```python
from build123d import *

# Parameters (mm, degrees)
SKETCH2_R          = 70
CUT_EXTRUDE1_DEPTH = 10
SKETCH3_R          = 20
CUT_EXTRUDE2_DEPTH = 121
SKETCH4_W          = 19.454924149
SKETCH4_H          = 15
CUT_EXTRUDE3_DEPTH = 121


with BuildPart() as part:
    # Sketch1 → Revolve1 (revolve)
    with BuildSketch(Plane.XY):
        Polygon((0, 65), (160, 65), (160, 40), (110, 40), (110, -40), (160, -40), (160, -65), (0, -65), align=None)
    revolve(axis=Axis((0, 93.810810811, 0), (0, -1, 0)))

    # Sketch2 → Cut-Extrude1 (cut)
    with BuildSketch(Plane(origin=(0, 65, 0), x_dir=(1, 0, 0), z_dir=(0, 1, 0))):
        Circle(SKETCH2_R)
    cut_extrude1 = extrude(amount=-CUT_EXTRUDE1_DEPTH, mode=Mode.SUBTRACT)

    # Mirror1: Cut-Extrude1 across plane
    add(cut_extrude1.mirror(Plane.ZX), mode=Mode.SUBTRACT)

    # Sketch3 → Cut-Extrude2 (cut, through all)
    with BuildSketch(Plane(origin=(0, 55, 0), x_dir=(1, 0, 0), z_dir=(0, 1, 0))):
        Circle(SKETCH3_R)
    extrude(amount=-CUT_EXTRUDE2_DEPTH, mode=Mode.SUBTRACT)

    # Sketch4 → Cut-Extrude3 (cut, through all)
    with BuildSketch(Plane(origin=(0, 55, 0), x_dir=(1, 0, 0), z_dir=(0, 1, 0))):
        with Locations((15.272537926, 0)):
            Rectangle(SKETCH4_W, SKETCH4_H)
    extrude(amount=-CUT_EXTRUDE3_DEPTH, mode=Mode.SUBTRACT)


solid = part.part
```
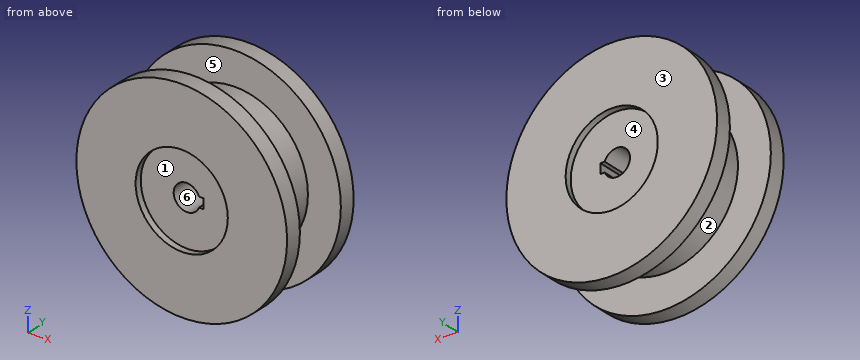
Build history of the part. All positions in model axes, mm. Face numbers are marked on the shaded views. A direction names the side the tool comes from. Round coordinates to 2 decimals unless told otherwise and drop trailing zeros. Write each loop counter-clockwise with the first axis right and the second up, starting at its lowest first coordinate (ties: lowest second). Pieces come first, ordered by that corner, then holes.
1) Band-saw the part on C-C, the plane y = 33. List the corners of the cut face in (x, z), and give its area (3 significant figures).
2) Band-saw the part on A-A, the plane z = 0. List the corners of the cut face in (x, y), and give its area (4 significant figures).
3) Drill centre lines: probe 1 along Y at (x, z) = (-85, 125); probe 2 along Z at (x, y) = (0, 60.75); probe 3 along Y at (x, z) = (-33.5, -8.5). Where is each one in solid material? Low to high.
4) Mould opens along Y. For the marked faces 1, 2 and 3 say: +Y half, -Y half, draft (parallel to the pull), parting line (faces both ways), or undercut.
5) 3-axis set-ups, long thin cutter, end or side, ignore diameter. For the marked faces 4, 5 and 6: which of +Z, -Z, +X, -X, +Y, -Y reach the whole face in a straight line?
6) Band-saw the part on B-B, the plane x = 0. List the corners of the cut face in (y, z), and give its area (3 significant figures).
7) Pin check, flat tips, straight feed: pin 1 (6 mm diameter, centred on y = 33.5, z = -48, fed in from +X); pin 2 (4 mm diameter, centred on x = -68.5, y = -11, fed in from -Z); pin 3 (2 mm diameter, centred on x = 52.5, y = -35.5, fed in from -Z). Stop position of each tip, or through.
8) Band-saw the part on D-D, the plane z = 38. List the corners of the cut face in (x, y).
Ans:
1. outline: circle Ø220 at (0, 0); hole (18.54, -7.5) - (25, -7.5) - (25, 7.5) - (18.54, 7.5) arc R20 ccw (long way) to start
1. area: 36,700 mm2
2. outline: (-160, -65) - (-70, -65) - (-70, -55) - (-20, -55) - (-20, 55) - (-70, 55) - (-70, 65) - (-160, 65) - (-160, 40) - (-110, 40) - (-110, -40) - (-160, -40) - close; (25, -55) - (70, -55) - (70, -65) - (160, -65) - (160, -40) - (110, -40) - (110, 40) - (160, 40) - (160, 65) - (70, 65) - (70, 55) - (25, 55) - close
2. area: 25,850 mm2
3. probe 1: y = -65 to -40, 40 to 65
3. probe 2: z = -160 to -70, 70 to 160
3. probe 3: y = -55 to 55
4. face 1: -Y half
4. face 2: undercut
4. face 3: +Y half
5. face 4: +Y
5. face 5: none
5. face 6: +Y, -Y
6. outline: (-65, -160) - (-40, -160) - (-40, -110) - (40, -110) - (40, -160) - (65, -160) - (65, -70) - (55, -70) - (55, -20) - (-55, -20) - (-55, -70) - (-65, -70) - close; (-65, 70) - (-55, 70) - (-55, 20) - (55, 20) - (55, 70) - (65, 70) - (65, 160) - (40, 160) - (40, 110) - (-40, 110) - (-40, 160) - (-65, 160) - close
6. area: 26,400 mm2
7. pin 1: stops at x = 100.37
7. pin 2: stops at z = -87.62
7. pin 3: stops at z = -97.2
8. outline: (-155.42, -65) - (-58.79, -65) - (-58.79, -55) - (58.79, -55) - (58.79, -65) - (155.42, -65) - (155.42, -40) - (103.23, -40) - (103.23, 40) - (155.42, 40) - (155.42, 65) - (58.79, 65) - (58.79, 55) - (-58.79, 55) - (-58.79, 65) - (-155.42, 65) - (-155.42, 40) - (-103.23, 40) - (-103.23, -40) - (-155.42, -40) - close
